Source: CAD feature listing. Evaluate the final solid. Frame: model axes, mm. A direction names the side the tool comes from. Coordinates: 2 decimals unless noted, no trailing zeros. Loops run counter-clockwise (first coordinate to the right, second up) from the corner with the lowest first, then second, coordinate; pieces in that order, holes last. Notation, with made-up numbers: M -38,-19 L 4,-19 A18 ccw 4,-7 Z; hole C 32.5,-37.75 d1. An arc over 180 degrees is marked long. One line per question, with ' | ' between items. Start each with the question number.
1. Pin query (flat end, axial travel): P1, Ø4, axis at x = -7.5, y = -3, coming from the -Z side; P2, Ø12, axis at x = 14, z = -8.5, coming from the -Y side; P3, Ø12, axis at x = 9.5, z = 5, coming from the -Y side; P4, Ø2, axis at x = 15.5, y = 5, coming from the +Z side. Return the tip coordinate at first contact, or that it passes through.
2. Section query B-B, the plane z = 0. Output: boundary loops of the cut face in (x, y).
3. Section query A-A, the plane x = 0. Output: boundary loops of the cut face in (y, z).
4. Mould query, pull axis Z, two halves, no side actions, for faces 1 (the flat face through (20, 1, 0)), 2 (the flat face through (0, 1, 20)), 3 (the flat face through (-4, 3, 4)). Classes: pulls with the +Z half, pulls with the -Z half, needs draft (parallel to the pull), parting line crosses it, or undercut.
5. Section query C-C, the plane y = 2.5. Output: boundary loops of the cut face in (x, z), and give its area (3 significant figures).
6. Access query for faces 4 (the cylindrical face through (15.52, 4.53, -14.17)), 5 (the flat face through (-9, 0, 0)), 6 (the flat face through (5, -4, 2)). Directions: +Z, -Z, +X, -X, +Y, -Y. A direction counts if a zero-diameter tool reaches every point of the face in a straight line with its end or side. Return the directions, or none.
7. Ray query, probe 1 along X at (y, z) = (1.25, 0); probe 2 along X at (y, z) = (-2, 0). Return the intervals inside material, ascending.
8. Section query D-D, the plane z = 12.7. Output: boundary loops of the cut face in (x, y).
```python
from build123d import *

# Parameters (mm, degrees)
EXTRUDE_1_DEPTH     = 3
SKETCH_2_R          = 3.18
EXTRUDE_2_DEPTH     = 3.1
SKETCH_3_R          = 5
CUT_EXTRUDE_1_DEPTH = 3.1
SKETCH_4_R          = 7.5
SKETCH_4_R_2        = 5
EXTRUDE_3_DEPTH     = 4


with BuildPart() as part:
    # 草图1 → 凸台-拉伸1 (new body)
    with BuildSketch(Plane(origin=(0, 0, 0), x_dir=(1, 0, 0), z_dir=(0, 1, 0))):
        with BuildLine():
            Line((-10, 20), (10, 20))
            ThreePointArc((10, 20), (17.071067812, 17.071067812), (20, 10))
            Line((20, 10), (20, -10))
            ThreePointArc((20, -10), (17.071067812, -17.071067812), (10, -20))
            Line((10, -20), (-10, -20))
            ThreePointArc((-10, -20), (-17.071067812, -17.071067812), (-20, -10))
            Line((-20, -10), (-20, 10))
            ThreePointArc((-20, 10), (-17.071067812, 17.071067812), (-10, 20))
        make_face()
    extrude(amount=EXTRUDE_1_DEPTH)

    # 草图2 → 凸台-拉伸2 (add)
    with BuildSketch(Plane(origin=(0, 3, 0), x_dir=(1, 0, 0), z_dir=(0, 1, 0))):
        with Locations(Location((12.7, 12.7, 0), (0, 0, 90))):
            Circle(SKETCH_2_R)
        with Locations(Location((12.7, -12.7, 0), (0, 0, 90))):
            Circle(SKETCH_2_R)
        with Locations(Location((-12.7, -12.7, 0), (0, 0, 90))):
            Circle(SKETCH_2_R)
        with Locations(Location((-12.7, 12.7, 0), (0, 0, 90))):
            Circle(SKETCH_2_R)
    extrude(amount=EXTRUDE_2_DEPTH)

    # 草图3 → 切除-拉伸1 (cut)
    with BuildSketch(Plane(origin=(0, 3, 0), x_dir=(1, 0, 0), z_dir=(0, 1, 0))):
        with Locations(Location((0, 0, 0), (0, 0, 270))):
            Circle(SKETCH_3_R)
    extrude(amount=-CUT_EXTRUDE_1_DEPTH, mode=Mode.SUBTRACT)

    # 草图4 → 凸台-拉伸3 (add)
    with BuildSketch(Plane.XZ):
        with Locations(Location((0, 0, 0), (0, 0, 90))):
            Circle(SKETCH_4_R)
        with Locations(Location((0, 0, 0), (0, 0, 90))):
            Circle(SKETCH_4_R_2, mode=Mode.SUBTRACT)
    extrude(amount=EXTRUDE_3_DEPTH)


solid = part.part
```
Taken from the geometry:
1) P1: z = -5.1 | P2: y = 0 | P3: y = -4 | P4: z = 15.32
2) outline: M -20,0 L -7.5,0 L -7.5,-4 L -5,-4 L -5,3 L -20,3 Z; M 5,-4 L 7.5,-4 L 7.5,0 L 20,0 L 20,3 L 5,3 Z
3) outline: M -4,-7.5 L 0,-7.5 L 0,-20 L 3,-20 L 3,-5 L -4,-5 Z; M -4,5 L 3,5 L 3,20 L 0,20 L 0,7.5 L -4,7.5 Z
4) face 1: needs draft | face 2: pulls with the +Z half | face 3: undercut
5) outline: M -20,-10 A10 ccw -10,-20 L 10,-20 A10 ccw 20,-10 L 20,10 A10 ccw 10,20 L -10,20 A10 ccw -20,10 Z; hole C 0,0 d10 | area: 1,440 mm^2
6) face 4: +Y | face 5: -Y | face 6: +Z, -Z, +X, -X, -Y
7) probe 1: -20 to -5, 5 to 20 | probe 2: -7.5 to -5, 5 to 7.5
8) outline: M -19.63,0 L 19.63,0 L 19.63,3 L 15.88,3 L 15.88,6.1 L 9.52,6.1 L 9.52,3 L -9.52,3 L -9.52,6.1 L -15.88,6.1 L -15.88,3 L -19.63,3 Z
